from build123d import *

# Parameters (mm, degrees)
SKETCH2_W           = 9.323493139
SKETCH2_H           = 24.035794238
BOSS_EXTRUDE1_DEPTH = 4


with BuildPart() as part:
    # Sketch2 → Boss-Extrude1 (new body)
    with BuildSketch(Plane.XY):
        with Locations((-0.028670292, 7.569333036)):
            Rectangle(SKETCH2_W, SKETCH2_H)
        with BuildLine():
            Line((2.42, 18.53), (-2.42, 18.53))
            Line((-2.42, 18.53), (-3.42, 1.411949008))
            ThreePointArc((-3.42, 1.411949008), (0, -3.7), (3.42, 1.411949008))
            Line((3.42, 1.411949008), (2.42, 18.53))
        make_face(mode=Mode.SUBTRACT)
    extrude(amount=BOSS_EXTRUDE1_DEPTH)


solid = part.part
The listing builds one solid part. Answer for the finished solid, in the listing's coordinates (mm). A direction names the side the tool comes from. Coordinates: 2 decimals unless noted, no trailing zeros. Write each loop counter-clockwise with the first axis right and the second up, starting at its lowest first coordinate (ties: lowest second). Pieces come first, ordered by that corner, then holes. Notation, with made-up numbers: (8, 21) - (16, 21) arc R5 cw to (16, 29) - close; hole circle Ø4 at (-13, 24.25). An arc over 180 degrees is marked (long way). Put each result on its own line as item: value.
1. The part is cut by section C-C on x = 0. Give the vertices of the cut face in (y, z), plus the area to 3 significant figures.
Answer sheet:
outline: (-4.45, 0) - (-3.7, 0) - (-3.7, 4) - (-4.45, 4) - close; (18.53, 0) - (19.59, 0) - (19.59, 4) - (18.53, 4) - close
area: 7.22 mm^2
2. A tool of negligible diameter and unlimited length cuts with its end or side. For faces 4 (the face through (-3.2, 10.3, 0)), 5 (the face through (-2.913, 10.091, 1.972)), from which of +Z, -Z, +X, -X, +Y, -Y can it reach the whole face along a straight path? Write none if from no direction.
Answer sheet:
face 4: -Z, +X, -X, +Y, -Y
face 5: +Z, -Z
3. The part is cut by section B-B on z = 3.3. Give the vertices of the cut face in (x, y), plus the area to 3 significant figures.
Answer sheet:
outline: (-4.69, -4.45) - (4.63, -4.45) - (4.63, 19.59) - (-4.69, 19.59) - close; hole (-3.42, 1.41) arc R3.7 ccw (long way) to (3.42, 1.41) - (2.42, 18.53) - (-2.42, 18.53) - close
area: 92.4 mm^2
4. Determine the mould class of faces 1 (the face through (-0.1, -3.7, 2)), 2 (the face through (4.633, 7, 2)), 3 (the face through (0, 19.587, 2)) for opening direction X: pulls with the +X half, pulls with the -X half, needs draft (parallel to the pull), parting line crosses it, or undercut.
Answer sheet:
face 1: undercut
face 2: pulls with the +X half
face 3: needs draft
5. The part is cut by section A-A on y = 0. Give the vertices of the cut face in (x, z), plus the area to 3 significant figures.
Answer sheet:
outline: (-4.69, 0) - (-3.7, 0) - (-3.7, 4) - (-4.69, 4) - close; (3.7, 0) - (4.63, 0) - (4.63, 4) - (3.7, 4) - close
area: 7.69 mm^2
6. Find the intervals of material crossed by line 1 along Y through (x, z) = (0, 2.75); line 2 along X through (y, z) = (1.5, 2.4); line 3 along X through (y, z) = (0, 2.05), in increasing order. Write a range as from..to.
Answer sheet:
line 1: y = -4.45..-3.7, 18.53..19.59
line 2: x = -4.69..-3.41, 3.41..4.63
line 3: x = -4.69..-3.7, 3.7..4.63
